Here's how the part is built. I have some questions about the finished solid (model axes, mm). Face numbers are marked on the shaded views. A direction names the side the tool comes from. Give positions to 0.01 mm unless a question says otherwise; leave off trailing zeros. Order: outer loops, then holes, each group sorted by start corner. A loop starts at its lowest first (then second) coordinate and runs counter-clockwise, first axis right, second up.
from build123d import *

# Parameters (mm, degrees)
FILLET_1_R          = 0.2
CHAMFER_1_SIZE      = 0.3
SKETCH_3_W          = 0.5
SKETCH_3_H          = 0.25
CUT_EXTRUDE_1_DEPTH = 2


with BuildPart() as part:
    # 草图1 → 旋转1 (revolve)
    with BuildSketch(Plane.XY):
        Polygon((-11.75, 0), (-11.75, 3.5), (-8.25, 3.5), (-8.25, 2), (5.75, 2), (5.75, 1.5), (11.75, 1.5), (11.75, 0), align=None)
    revolve(axis=Axis((-11.75, 0, 0), (1, 0, 0)))

    # 圆角1
    fillet_1_edges = [part.edges().sort_by_distance(p)[0] for p in [
        (-8.25, -3.5, 0),
        (-11.75, -3.5, 0),
    ]]
    fillet(fillet_1_edges, radius=FILLET_1_R)

    # 倒角1
    chamfer_1_edges = [part.edges().sort_by_distance(p)[0] for p in [
        (11.75, -1.5, 0),
    ]]
    chamfer(chamfer_1_edges, length=CHAMFER_1_SIZE)

    # 草图3 → 切除-旋转1 (revolve, cut)
    with BuildSketch(Plane.XY):
        with Locations((6, 1.375)):
            Rectangle(SKETCH_3_W, SKETCH_3_H)
    revolve(axis=Axis((5.75, 0, 0), (1, 0, 0)), mode=Mode.SUBTRACT)

    # 草图4 → 切除-拉伸1 (cut)
    with BuildSketch(Plane.ZY.offset(11.75)):
        Polygon((1.732050808, 0), (0.866025404, 1.5), (-0.866025404, 1.5), (-1.732050808, 0), (-0.866025404, -1.5), (0.866025404, -1.5), align=None)
    extrude(amount=-CUT_EXTRUDE_1_DEPTH, mode=Mode.SUBTRACT)


solid = part.part
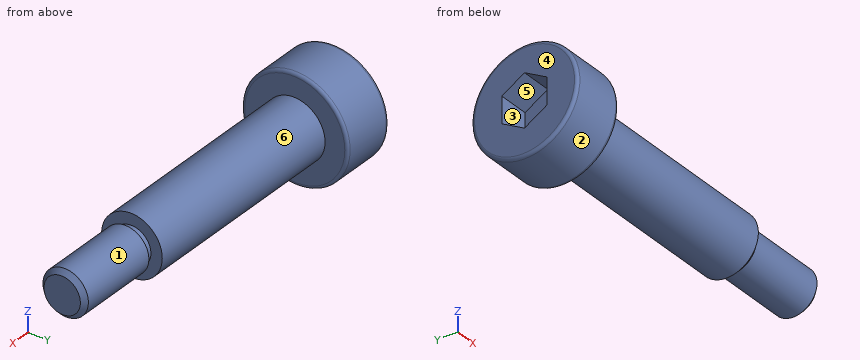
Q1. If we section it at A-A on z = 0: List the corners of the cut face in (x, y) for me, plus the area to 3 significant figures.
Filled sheet:
outline: (-11.75, -3.3) arc R0.2 ccw to (-11.55, -3.5) - (-8.45, -3.5) arc R0.2 ccw to (-8.25, -3.3) - (-8.25, -2) - (5.75, -2) - (5.75, -1.25) - (6.25, -1.25) - (6.25, -1.5) - (11.45, -1.5) - (11.75, -1.2) - (11.75, 1.2) - (11.45, 1.5) - (6.25, 1.5) - (6.25, 1.25) - (5.75, 1.25) - (5.75, 2) - (-8.25, 2) - (-8.25, 3.3) arc R0.2 ccw to (-8.45, 3.5) - (-11.55, 3.5) arc R0.2 ccw to (-11.75, 3.3) - (-11.75, 1.5) - (-9.75, 1.5) - (-9.75, -1.5) - (-11.75, -1.5) - close
area: 92.1 mm2
Q2. Thinking about a two-plate mould opening in Y: for the marked faces 4, 5 and 6, which applies, released by +Y, released by -Y, zero draft, split by the parting line, or undercut?
Filled sheet:
face 4: zero draft
face 5: undercut
face 6: split by the parting line
Q3. If we section it at C-C on x = -9.5: List the corners of the cut face in (y, z) for me.
Filled sheet:
outline: circle Ø7 at (0, 0)
Q4. I need wall thicknesses on L1, parallel to X at y = -2, z = 2.5; L2, parallel to X at y = -0.75, z = 0.5; L3, parallel to Z at x = -4, y = -1. Which ranges of each line are inside material? Lowest first, please.
Filled sheet:
L1: x = -11.75 to -8.25
L2: x = -9.75 to 11.75
L3: z = -1.73 to 1.73
Q5. I'm going to push flat-ended pins straight in: P1, Ø1.5, axis at x = -1, y = 2.5, coming from the -Z side; P2, Ø1.5, axis at y = 0.5, z = 0.5, coming from the -X side; P3, Ø1.5, axis at x = -1.5, y = -2.5, coming from the +Z side. Where does each tip first touch, or does it pass through?
Filled sheet:
P1: stops at z = -0.97
P2: stops at x = -9.75
P3: stops at z = 0.97
Q6. If we section it at B-B on x = 7: List the corners of the cut face in (y, z) for me, plus the area to 3 significant figures.
Filled sheet:
outline: circle Ø3 at (0, 0)
area: 7.07 mm2
Q7. For the marked faces 1, 2 and 3, which set-ups out of +Z, -Z, +X, -X, +Y, -Y let a thin tool reach every point of the face, with its end or its side?
Filled sheet:
face 1: +X
face 2: +X, -X
face 3: -X
